Geometry: see drawing. Coordinates: mm, zero at the bounding-box minimum. A direction names the side the tool comes from. Give positions to 0.01 mm unless a question says otherwise; leave off trailing zeros. Loops run counter-clockwise (first coordinate to the right, second up) from the corner with the lowest first, then second, coordinate; pieces in that order, holes last. Notation, with made-up numbers: (13, 44) - (21, 44) arc R27 cw to (21, 75) - close; hole circle Ø7 at (40.25, 80.5). An arc over 180 degrees is marked (long way). Use CSV: the item, a comma, the result in double quotes. Start each with the question number.
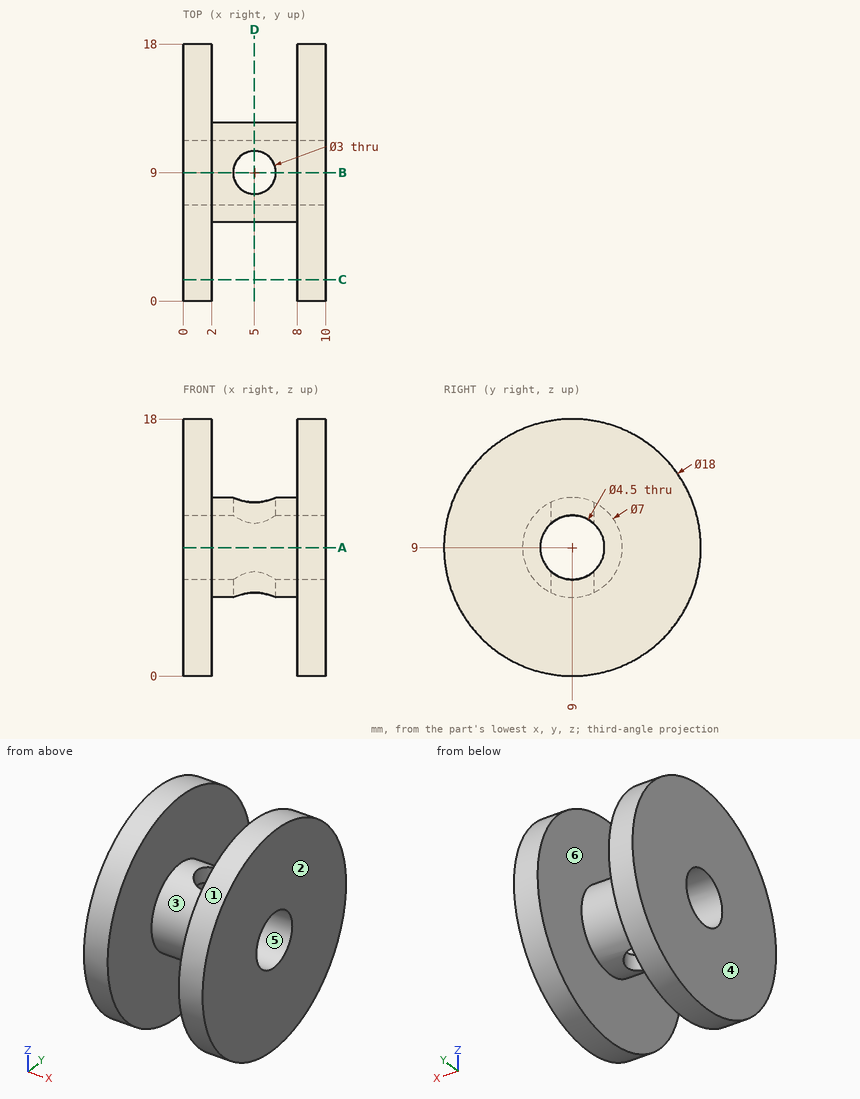
Item 1: Section D-D (x = 5). Output: boundary loops of the cut face in (y, z).
Item 2: Section B-B (y = 9). Output: boundary loops of the cut face in (x, z), plus the area to 3 significant figures.
Item 3: Pin query (flat end, axial travel): pin 1 Ø5 at (x, z) = (3.5, 6) entering from -Y; pin 2 Ø1.5 at (x, y) = (6.5, 9.5) entering from -Z; pin 3 Ø1.5 at (x, z) = (4, 8.5) entering from -Y; pin 4 Ø3 at (x, z) = (6, 14) entering from +Y (3 decimals). Return the tip coordinate at first contact, or that it passes through.
Item 4: Section C-C (y = 1.5). Output: boundary loops of the cut face in (x, z).
Item 5: Reachability of the marked faces 5 and 6 from +Z, -Z, +X, -X, +Y, -Y: full face, straight path, thin tool, end or side. Return the list, or none.
Item 6: Section A-A (z = 9). Output: boundary loops of the cut face in (x, y), plus the area to 3 significant figures.
Item 7: Mould query, pull axis X, two halves, no side actions, for the marked faces 1, 2, 3 and 4. Classes: pulls with the +X half, pulls with the -X half, needs draft (parallel to the pull), parting line crosses it, or undercut.
Item 8: Ray query, probe 1 along X at (y, z) = (6.5, 13.25); probe 2 along Y at (x, z) = (6.25, 9); probe 3 along X at (y, z) = (9, 5.95). Return the intervals inside material, ascending.
Outcome:
1,outline,"(7.5, 5.84) - (7.5, 7.32) arc R2.25 cw to (7.5, 10.68) - (7.5, 12.16) arc R3.5 ccw to start; (10.5, 5.84) arc R3.5 ccw to (10.5, 12.16) - (10.5, 10.68) arc R2.25 cw to (10.5, 7.32) - close"
2,outline,"(0, 0) - (2, 0) - (2, 5.5) - (3.5, 5.5) - (3.5, 6.75) - (0, 6.75) - close; (0, 11.25) - (3.5, 11.25) - (3.5, 12.5) - (2, 12.5) - (2, 18) - (0, 18) - close; (6.5, 5.5) - (8, 5.5) - (8, 0) - (10, 0) - (10, 6.75) - (6.5, 6.75) - close; (6.5, 11.25) - (10, 11.25) - (10, 18) - (8, 18) - (8, 12.5) - (6.5, 12.5) - close"
2,area,"61.5 mm2"
3,pin 1,"stops at y = 0.06"
3,pin 2,"stops at z = 5.5"
3,pin 3,"stops at y = 5.5"
3,pin 4,"passes through"
4,outline,"(0, 4.03) - (2, 4.03) - (2, 13.97) - (0, 13.97) - close; (8, 4.03) - (10, 4.03) - (10, 13.97) - (8, 13.97) - close"
5,face 5,"+X, -X"
5,face 6,"none"
6,outline,"(0, 0) - (2, 0) - (2, 5.5) - (8, 5.5) - (8, 0) - (10, 0) - (10, 6.75) - (0, 6.75) - close; (0, 11.25) - (10, 11.25) - (10, 18) - (8, 18) - (8, 12.5) - (2, 12.5) - (2, 18) - (0, 18) - close"
6,area,"69.0 mm2"
7,face 1,"needs draft"
7,face 2,"pulls with the +X half"
7,face 3,"undercut"
7,face 4,"pulls with the -X half"
8,probe 1,"x = 0 to 2, 8 to 10"
8,probe 2,"y = 5.5 to 6.75, 11.25 to 12.5"
8,probe 3,"x = 0 to 3.5, 6.5 to 10"
